Check sheet for the modelled part. Datum: model origin and axes. Units: mm. A direction names the side the tool comes from. Round coordinates to 2 decimals unless told otherwise and drop trailing zeros. Loops run counter-clockwise (first coordinate to the right, second up) from the corner with the lowest first, then second, coordinate; pieces in that order, holes last. Notation, with made-up numbers: (58, -39) - (103, -39) arc R24 ccw to (103, -3) - close; hole circle Ø3 at (21.25, 46.25). An arc over 180 degrees is marked (long way). Put each result on its own line as item: value. Start each with the question number.
```python
from build123d import *

# Parameters (mm, degrees)
F0_W     = 88.9
F0_H     = 88.9
F0_W_2   = 79.375
F0_H_2   = 79.375
F1_DEPTH = 63.5
F3_W     = 5.55625
F3_H     = 7.9375
F4_DEPTH = 88.901
F2_W     = 79.375
F2_H     = 25.4
F5_DEPTH = 88.901


with BuildPart() as f1:
    # F0 (on Top) → F1 (new body)
    with BuildSketch(Plane.XY):
        Rectangle(F0_W, F0_H)
        Rectangle(F0_W_2, F0_H_2, mode=Mode.SUBTRACT)
    extrude(amount=F1_DEPTH)

    # F3 (on face) → F4 (cut, through all)
    with BuildSketch(Plane(origin=(0, 44.45, 0), x_dir=(-1, 0, 0), z_dir=(0, 1, 0))):
        with Locations((2.778125, 50.8)):
            Rectangle(F3_W, F3_H)
        with Locations((-2.778125, 50.8)):
            Rectangle(F3_W, F3_H)
    extrude(amount=-F4_DEPTH, mode=Mode.SUBTRACT)

    # F2 (on face) → F5 (cut, through all)
    with BuildSketch(Plane(origin=(-44.45, 0, 0), x_dir=(0, -1, 0), z_dir=(-1, 0, 0))):
        with Locations((0, 50.8)):
            Rectangle(F2_W, F2_H)
    extrude(amount=-F5_DEPTH, mode=Mode.SUBTRACT)


solid = f1.part
```
Q1. Cross-section at B-B on y = 2. Enter the section's corners in (x, z), and give its area (3 significant figures).
Q2. Cross-section at D-D on z = 52. Enter the section's corners in (x, y), and give its area (3 significant figures).
Q3. Depth check by flat-ended pin: pin 1 Ø1.4 at (x, y) = (-0.5, -42.5) entering from -Z; pin 2 Ø2.5 at (x, y) = (-42, 19) entering from +Z; pin 3 Ø8 at (x, y) = (-5, -33) entering from +Z. Enter the tip coordinate at first touch or a pass-through.
Q4. Cross-section at A-A on x = -29. Enter the section's corners in (y, z), and give its area (3 significant figures).
Q5. Cross-section at C-C on z = 15.5. Enter the section's corners in (x, y), and give its area (3 significant figures).
Q6. Draft check along Y on faces 5 (the face through (39.688, -1, 19)), 6 (the face through (-1, -42, 63.5)), 7 (the face through (-1, 44.45, 31)). Enter one of: +Y half, -Y half, draft (parallel to the pull), parting line (faces both ways), or undercut.
Q7. Set-up check for faces 1 (the face through (-39.688, -1, 19)), 2 (the face through (0, -42, 54.769)), 3 (the face through (-42, 1, 38.1)), 4 (the face through (44.45, -1, 17)): record each of +Z, -Z, +X, -X, +Y, -Y from which the full face is reachable in a straight line by a thin tool's end or side.
Q8. Material ranges on line 1 (Y direction, x = -10.5, z = 3.5), recorded low to high. Write a range as from..to.
Answer list:
1. outline: (-44.45, 0) - (-39.69, 0) - (-39.69, 38.1) - (-44.45, 38.1) - close; (39.69, 0) - (44.45, 0) - (44.45, 38.1) - (39.69, 38.1) - close
1. area: 363 mm2
2. outline: (-44.45, -44.45) - (-5.56, -44.45) - (-5.56, -39.69) - (-44.45, -39.69) - close; (-44.45, 39.69) - (-5.56, 39.69) - (-5.56, 44.45) - (-44.45, 44.45) - close; (5.56, -44.45) - (44.45, -44.45) - (44.45, -39.69) - (5.56, -39.69) - close; (5.56, 39.69) - (44.45, 39.69) - (44.45, 44.45) - (5.56, 44.45) - close
2. area: 741 mm2
3. pin 1: stops at z = 0
3. pin 2: stops at z = 38.1
3. pin 3: passes through
4. outline: (-44.45, 0) - (-39.69, 0) - (-39.69, 63.5) - (-44.45, 63.5) - close; (39.69, 0) - (44.45, 0) - (44.45, 63.5) - (39.69, 63.5) - close
4. area: 605 mm2
5. outline: (-44.45, -44.45) - (44.45, -44.45) - (44.45, 44.45) - (-44.45, 44.45) - close; hole (-39.69, -39.69) - (39.69, -39.69) - (39.69, 39.69) - (-39.69, 39.69) - close
5. area: 1,600 mm2
6. face 5: undercut
6. face 6: draft
6. face 7: +Y half
7. face 1: +Z, -Z
7. face 2: +Y, -Y
7. face 3: +Z, +X, -X
7. face 4: +Z, -Z, +X, +Y, -Y
8. line 1: y = -44.45..-39.69, 39.69..44.45
